Can you work these out from the model? Positions are in its coordinate system, mm. A direction names the side the tool comes from. Give positions to 0.01 mm unless a question says otherwise; leave off trailing zeros. Write each loop counter-clockwise with the first axis right and the second up, starting at its lowest first coordinate (ties: lowest second). Pieces come first, ordered by that corner, then holes.
```python
from build123d import *

# Parameters (mm, degrees)
EXTRUDE_1_DEPTH      = 3
FILLET_1_R           = 0.5
EXTRUDE_2_DEPTH      = 12
FILLET_2_R           = 1.5
SKETCH_4_W           = 2
SKETCH_4_H           = 6
CUT_EXTRUDE_1_DEPTH  = 4
EXTRUDE_3_DEPTH      = 2
EXTRUDE_3_DEPTH_BACK = 4


with BuildPart() as part:
    # Sketch 2 → Extrude 1 (new body)
    with BuildSketch(Plane.XY):
        with BuildLine():
            Line((0, 0), (-7.5, 0))
            ThreePointArc((-7.5, 0), (-8.349754016, -0.263910152), (-8.900496416, -0.96277585))
            add(Edge.make_bspline(
                [(-8.900496416, -0.96277585), (-9.890641619, -3.543997872), (-11.090476147, -5.889739255), (-12.5, -8)],
                knots=[0.057327247, 0.057327247, 0.057327247, 0.057327247, 0.826256539, 0.826256539, 0.826256539, 0.826256539], degree=3))
            Line((-12.5, -8), (-16.55, -8))
            ThreePointArc((-16.55, -8), (-17.610660172, -8.439339828), (-18.05, -9.5))
            Line((-18.05, -9.5), (-18.05, -25.75))
            Line((-18.05, -25.75), (0, -25.75))
            Line((0, -25.75), (0, -5.55))
            Line((0, -5.55), (-6, -5.55))
            ThreePointArc((-6, -5.55), (-7.55, -4), (-6, -2.45))
            Line((-6, -2.45), (0, -2.45))
            Line((0, -2.45), (0, 0))
        make_face()
        with BuildLine():
            Line((7.5, 0), (0, 0))
            Line((0, 0), (0, -2.45))
            Line((0, -2.45), (6, -2.45))
            ThreePointArc((6, -2.45), (7.55, -4), (6, -5.55))
            Line((6, -5.55), (0, -5.55))
            Line((0, -5.55), (0, -25.75))
            Line((0, -25.75), (18.05, -25.75))
            Line((18.05, -25.75), (18.05, -9.5))
            ThreePointArc((18.05, -9.5), (17.610660172, -8.439339828), (16.55, -8))
            Line((16.55, -8), (12.5, -8))
            add(Edge.make_bspline(
                [(8.900496416, -0.96277585), (9.890641619, -3.543997872), (11.090476147, -5.889739255), (12.5, -8)],
                knots=[0.057327247, 0.057327247, 0.057327247, 0.057327247, 0.826256539, 0.826256539, 0.826256539, 0.826256539], degree=3))
            ThreePointArc((8.900496416, -0.96277585), (8.349754016, -0.263910152), (7.5, 0))
        make_face()
        with BuildLine():
            Line((18.05, -25.75), (0, -25.75))
            Line((0, -25.75), (0, -45.95))
            Line((0, -45.95), (6, -45.95))
            ThreePointArc((6, -45.95), (7.55, -47.5), (6, -49.05))
            Line((6, -49.05), (0, -49.05))
            Line((0, -49.05), (0, -51.5))
            Line((0, -51.5), (7.5, -51.5))
            ThreePointArc((7.5, -51.5), (8.349754016, -51.236089848), (8.900496416, -50.53722415))
            add(Edge.make_bspline(
                [(8.900496416, -50.53722415), (9.890641619, -47.956002128), (11.090476147, -45.610260745), (12.5, -43.5)],
                knots=[0.057327247, 0.057327247, 0.057327247, 0.057327247, 0.826256539, 0.826256539, 0.826256539, 0.826256539], degree=3))
            Line((12.5, -43.5), (16.55, -43.5))
            ThreePointArc((16.55, -43.5), (17.610660172, -43.060660172), (18.05, -42))
            Line((18.05, -42), (18.05, -25.75))
        make_face()
        with BuildLine():
            Line((0, -45.95), (0, -25.75))
            Line((0, -25.75), (-18.05, -25.75))
            Line((-18.05, -25.75), (-18.05, -42))
            ThreePointArc((-18.05, -42), (-17.610660172, -43.060660172), (-16.55, -43.5))
            Line((-16.55, -43.5), (-12.5, -43.5))
            add(Edge.make_bspline(
                [(-8.900496416, -50.53722415), (-9.890641619, -47.956002128), (-11.090476147, -45.610260745), (-12.5, -43.5)],
                knots=[0.057327247, 0.057327247, 0.057327247, 0.057327247, 0.826256539, 0.826256539, 0.826256539, 0.826256539], degree=3))
            ThreePointArc((-8.900496416, -50.53722415), (-8.349754016, -51.236089848), (-7.5, -51.5))
            Line((-7.5, -51.5), (0, -51.5))
            Line((0, -51.5), (0, -49.05))
            Line((0, -49.05), (-6, -49.05))
            ThreePointArc((-6, -49.05), (-7.55, -47.5), (-6, -45.95))
            Line((-6, -45.95), (0, -45.95))
        make_face()
    extrude(amount=EXTRUDE_1_DEPTH)

    # Fillet 1
    fillet_1_edges = [part.edges().sort_by_distance(p)[0] for p in [
        (12.5, -8, 1.5),
        (12.5, -43.5, 1.5),
        (-12.5, -43.5, 1.5),
        (-12.5, -8, 1.5),
    ]]
    fillet(fillet_1_edges, radius=FILLET_1_R)

    # Sketch 3 → Extrude 2 (add)
    with BuildSketch(Plane.XY.offset(3)):
        with BuildLine():
            Line((0, -8), (16.55, -8))
            ThreePointArc((16.55, -8), (17.610660172, -8.439339828), (18.05, -9.5))
            Line((18.05, -9.5), (18.05, -42))
            ThreePointArc((18.05, -42), (17.610660172, -43.060660172), (16.55, -43.5))
            Line((16.55, -43.5), (14.659338555, -43.5))
            Line((14.659338555, -43.5), (-16.55, -43.5))
            ThreePointArc((-16.55, -43.5), (-17.610660172, -43.060660172), (-18.05, -42))
            Line((-18.05, -42), (-18.05, -25.75))
            Line((-18.05, -25.75), (-18.05, -9.5))
            ThreePointArc((-18.05, -9.5), (-17.610660172, -8.439339828), (-16.55, -8))
            Line((-16.55, -8), (0, -8))
        make_face()
    extrude(amount=EXTRUDE_2_DEPTH)

    # Fillet 2
    fillet_2_edges = [part.edges().sort_by_distance(p)[0] for p in [
        (0, -8, 15),
        (-17.610660172, -8.439339828, 15),
        (-18.05, -25.75, 15),
        (-17.610660172, -43.060660172, 15),
        (0, -43.5, 15),
        (17.610660172, -43.060660172, 15),
        (18.05, -25.75, 15),
        (17.610660172, -8.439339828, 15),
    ]]
    fillet(fillet_2_edges, radius=FILLET_2_R)

    # Sketch 4 → Cut-Extrude 1 (cut)
    with BuildSketch(Plane.ZY.offset(18.05)):
        with Locations((7.5, -25.75)):
            Rectangle(SKETCH_4_W, SKETCH_4_H)
    extrude(amount=-CUT_EXTRUDE_1_DEPTH, mode=Mode.SUBTRACT)

    # Sketch 4_3 → Extrude 3 (add, two sides: drawn at the far end of the back side and taken through both)
    with BuildSketch(Plane.ZY.offset(18.05).offset(-EXTRUDE_3_DEPTH_BACK)):
        Polygon((8.25, -28.5), (8.25, -25.75), (7.5, -25.75), (6.75, -25.75), (6.75, -28.5), align=None)
    extrude(amount=EXTRUDE_3_DEPTH + EXTRUDE_3_DEPTH_BACK)


solid = part.part
```
1) Please list where these lines run through material, in increasing order: L1, parallel to X at y = -24, z = 3.25; L2, parallel to Z at x = 7, y = -5.5; L3, parallel to Y at x = 8.5, z = 10.75.
Values follow:
L1: x = -18.05 to 18.05
L2: z = 0 to 3
L3: y = -43.5 to -8
2) Suppose I cut it at A-A on x = -3. Write out the boundary of the cut face in (y, z), plus the area to 3 significant figures.
Values follow:
outline: (-51.5, 0) - (-49.05, 0) - (-49.05, 3) - (-51.5, 3) - close; (-45.95, 0) - (-5.55, 0) - (-5.55, 3) - (-8, 3) - (-8, 13.5) arc R1.5 ccw to (-9.5, 15) - (-42, 15) arc R1.5 ccw to (-43.5, 13.5) - (-43.5, 3) - (-45.95, 3) - close; (-2.45, 0) - (0, 0) - (0, 3) - (-2.45, 3) - close
area: 561 mm2
3) Suppose I cut it at D-D on z = 2. State how many separate pieces and enclosed holes the cut face has, plus the area to 3 significant figures.
Values follow:
separate pieces: 1
enclosed holes: 2
area: 1,520 mm2
4) Suppose I cut it at C-C on y = -39. Write out the boundary of the cut face in (x, z), plus the area to 3 significant figures.
Values follow:
outline: (-18.05, 0) - (18.05, 0) - (18.05, 13.5) arc R1.5 ccw to (16.55, 15) - (-16.55, 15) arc R1.5 ccw to (-18.05, 13.5) - close
area: 541 mm2
5) For faces 1 (the face through (7.55, -3.97, 1.48)), 2 (the face through (-20.05, -27, 7)), 3 (the face through (-17.6, -43.07, 6.66)), 4 (the face through (-16, -22.75, 7)), 5 (the face through (-0.2, -45.7, 3)), which set-ups out of +Z, -Z, +X, -X, +Y, -Y let a thin tool reach every point of the face, with its end or its side?
Values follow:
face 1: +Z, -Z
face 2: +Z, -Z, -X, +Y, -Y
face 3: +Z, -Z, -X, -Y
face 4: -X
face 5: +Z, +X, -X, -Y
6) Suppose I cut it at B-B on z = 11.5. Write out the boundary of the cut face in (x, y), plus the area to 3 significant figures.
Values follow:
outline: (-18.05, -42) arc R1.5 ccw to (-16.55, -43.5) - (16.55, -43.5) arc R1.5 ccw to (18.05, -42) - (18.05, -9.5) arc R1.5 ccw to (16.55, -8) - (-16.55, -8) arc R1.5 ccw to (-18.05, -9.5) - close
area: 1,280 mm2
7) If we mould it in two halves opening along Y, with no side actions, what happens to faces 6 (the face through (0, -25, 0)), 7 (the face through (8.4, -0.3, 1.5)), 8 (the face through (-17, -28.5, 7))? For each: +Y half, -Y half, draft (parallel to the pull), parting line (faces both ways), or undercut.
Values follow:
face 6: draft
face 7: +Y half
face 8: undercut
8) For pin 1 Ø0.6 at (x, z) = (-16.5, 7) entering from +Y; pin 2 Ø1.6 at (x, z) = (-17.5, 7.5) entering from -Y; pin 3 Ø6.5 at (x, y) = (-3, -3) entering from +Z, each with a flat end and sliding along its axis, tell me the tip position at first contact or that it passes through.
Values follow:
pin 1: stops at y = -8
pin 2: stops at y = -43.49
pin 3: stops at z = 3
